Could you check a few things on this model? Use its own coordinates, in mm. Give positions to 0.01 mm unless a question says otherwise; leave off trailing zeros. Loops run counter-clockwise (first coordinate to the right, second up) from the corner with the lowest first, then second, coordinate; pieces in that order, holes last. Notation, with made-up numbers: M 62.25,34 L 107.25,34 A19 cw 107.25,56 Z; hole C 70,77.25 d2. An arc over 180 degrees is marked long. Return JSON: item names as keys, results as strings. Group by question number.
1. If we section it at A-A (z = -0.05): Write out the boundary of the cut face in (x, y).
2. If we section it at C-C (x = 1.5): Write out the boundary of the cut face in (y, z).
3. If we section it at B-B (y = -8): Write out the boundary of the cut face in (x, z).
4. Please list where these lines run through material, in increasing order: line 1 (Y direction, x = 0.75, z = -0.05); line 2 (X direction, y = -7.5, z = -0.1).
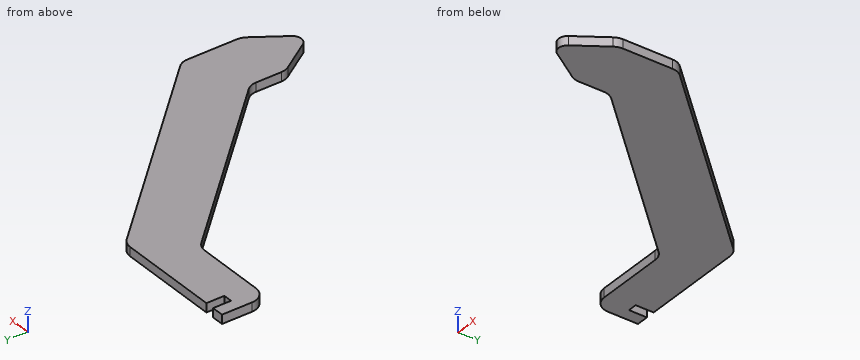
```python
from build123d import *

# Parameters (mm, degrees)
BOSS_EXTRUDE1_DEPTH = 0.15
FILLET1_R           = 0.3
FILLET2_R           = 0.5


with BuildPart() as part:
    # Sketch1 → Boss-Extrude1 (new, symmetric)
    with BuildSketch(Plane.XY):
        Polygon((0, 0), (0.4, 0), (0.4, -0.6), (0.7, -0.6), (0.7, 0), (4.332844343, 0), (10.55, -6.5), (10.55, -8.5), (9.55, -10), (8.55, -8.5), (8.55, -7.302492649), (3, -1.5), (0, -1.5), align=None)
    extrude(amount=BOSS_EXTRUDE1_DEPTH, both=True)

    # Fillet1
    fillet1_edges = [part.edges().sort_by_distance(p)[0] for p in [
        (9.55, -10, 0),
    ]]
    fillet(fillet1_edges, radius=FILLET1_R)

    # Fillet2
    fillet2_edges = [part.edges().sort_by_distance(p)[0] for p in [
        (4.332844343, 0, 0),
        (10.55, -6.5, 0),
        (10.55, -8.5, 0),
        (8.55, -8.5, 0),
        (8.55, -7.302492649, 0),
        (3, -1.5, 0),
        (0, -1.5, 0),
    ]]
    fillet(fillet2_edges, radius=FILLET2_R)


solid = part.part
```
Answer:
{
 "1": {"outline": "M 0,-1 A0.5 ccw 0.5,-1.5 L 2.79,-1.5 A0.5 cw 3.15,-1.65 L 8.41,-7.16 A0.5 cw 8.55,-7.5 L 8.55,-8.35 A0.5 ccw 8.63,-8.63 L 9.3,-9.63 A0.3 ccw 9.8,-9.63 L 10.47,-8.63 A0.5 ccw 10.55,-8.35 L 10.55,-6.7 A0.5 ccw 10.41,-6.36 L 4.48,-0.15 A0.5 ccw 4.12,0 L 0.7,0 L 0.7,-0.6 L 0.4,-0.6 L 0.4,0 L 0,0 Z"},
 "2": {"outline": "M -1.5,-0.15 L 0,-0.15 L 0,0.15 L -1.5,0.15 Z"},
 "3": {"outline": "M 8.55,-0.15 L 10.55,-0.15 L 10.55,0.15 L 8.55,0.15 Z"},
 "4": {"line 1": "y = -1.5 to 0", "line 2": "x = 8.55 to 10.55"}
}
